Part model, mm, in its own coordinate system. A direction names the side the tool comes from. Round coordinates to 2 decimals unless told otherwise and drop trailing zeros. Write each loop counter-clockwise with the first axis right and the second up, starting at its lowest first coordinate (ties: lowest second). Pieces come first, ordered by that corner, then holes. Notation, with made-up numbers: M 28,19 L 32,19 A27 cw 32,44 Z; hole C 14.5,12.5 d7. An arc over 180 degrees is marked long. Answer as a JSON object with one key per item and string values. Group by question number.
1. Band-saw the part on B-B, the plane y = -76. Write the cut outline in (x, z), plus the area to 3 significant figures.
2. Two-plate mould, pull along Z, no slides. Class faces 1 (the face through (-557.59, 0.09, -6.7)), 2 (the face through (6, -2, 6.35)), 3 (the face through (-529.17, 0.089, 19.663)): +Z half, -Z half, draft (parallel to the pull), parting line (faces both ways), or undercut.
3. Drop flat-ended pins along their axis: pin 1 (6.5 mm diameter, centred on y = -54.5, z = 2.5, fed in from -X); pin 2 (6 mm diameter, centred on x = -98, z = 6.5, fed in from +Y); pin 3 (4 mm diameter, centred on x = 4, y = 30, fed in from +Z). Give the stop position or say it passes through.
4. Band-saw the part on C-C, the plane x = -351.5. Write the cut outline in (y, z).
5. Drill centre lines: line 1 (Z direction, x = -133.5, y = 1); line 2 (Z direction, x = -244.5, y = -3.5). Where is each one in solid material? Low to high. Write a range as from..to.
6. Band-saw the part on A-A, the plane x = -513. Count the separate pieces of the cut face and the enclosed holes in it, plus the area to 3 significant figures.
7. Which spindle directions (+Z, -Z, +X, -X, +Y, -Y) get a long thin tool onto all of the face, cutting with end or side? Do faces 4 (the face through (-521, -6.35, 25)), 5 (the face through (-521, 6.35, 25)), 6 (the face through (-528.791, 0.089, 85.426)). Say none if no direction does.
from build123d import *

# Parameters (mm, degrees)
F0_W      = 254
F0_H      = 12.7
F1_DEPTH  = 12.7
F3_DEPTH  = 558.8
F4_R      = 7.62
F6_DEPTH  = 12.7
F7_W      = 101.6
F7_H      = 12.7
F8_DEPTH  = 2.54
F10_DEPTH = 50.8


with BuildPart() as f1:
    # F0 (on Right) → F1 (new body)
    with BuildSketch(Plane.YZ):
        Rectangle(F0_W, F0_H)
    extrude(amount=F1_DEPTH)

    # F2 (on face) → F3 (join)
    with BuildSketch(Plane(origin=(0, 0, 0), x_dir=(0, -1, 0), z_dir=(-1, 0, 0))):
        with BuildLine():
            ThreePointArc((-6.84e-08, -6.35), (4.4901280364, -4.4901280847), (6.35, 0))
            ThreePointArc((6.35, 0), (4.4901280521, 4.4901280689), (-2.37e-08, 6.35))
            ThreePointArc((-2.37e-08, 6.35), (-6.35, 2.23e-08), (-6.84e-08, -6.35))
        make_face()
    extrude(amount=F3_DEPTH)

    # F4
    f4_edges = [f1.edges().sort_by_distance(p)[0] for p in [
        (6.35, -127, -6.35),
        (6.35, 127, -6.35),
    ]]
    fillet(f4_edges, radius=F4_R)

    # F5 (on Front) → F6 (cut, symmetric)
    with BuildSketch(Plane.XZ):
        Polygon((-541.0905659676, 6.7056384869), (-558.8, 6.7056384869), (-558.8, -7.6832813211), align=None)
    extrude(amount=F6_DEPTH, both=True, mode=Mode.SUBTRACT)

    # F7 (on face) → F8 (join)
    with BuildSketch(Plane(origin=(-218.4449745832, 0, 268.8552663249), x_dir=(0.7761139002, 0, 0.630592748), z_dir=(-0.630592748, 0, 0.7761139002))):
        with Locations((-388.1941093914, 0)):
            Rectangle(F7_W, F7_H)
    extrude(amount=F8_DEPTH)

    # F9 (on face) → F10 (join)
    with BuildSketch(Plane(origin=(-220.0466801631, 0, 270.8265956315), x_dir=(0.7761139002, 0, 0.630592748), z_dir=(-0.630592748, 0, 0.7761139002))):
        with BuildLine():
            ThreePointArc((-356.4441093914, -6.35), (-351.9539813308, -4.4901280605), (-350.0941093914, 0))
            ThreePointArc((-350.0941093914, 0), (-351.9539813308, 4.4901280605), (-356.4441093914, 6.35))
            ThreePointArc((-356.4441093914, 6.35), (-362.7941093914, 0), (-356.4441093914, -6.35))
        make_face()
    extrude(amount=F10_DEPTH)


solid = f1.part
Worked answers:
{
 "1": {"outline": "M 0,-6.35 L 12.7,-6.35 L 12.7,6.35 L 0,6.35 Z", "area": "161 mm^2"},
 "2": {"face 1": "-Z half", "face 2": "+Z half", "face 3": "undercut"},
 "3": {"pin 1": "stops at x = 0", "pin 2": "stops at y = 5.3", "pin 3": "stops at z = 6.35"},
 "4": {"outline": "C 0,0 d12.7"},
 "5": {"line 1": "z = -6.27..6.27", "line 2": "z = -5.3..5.3"},
 "6": {"separate pieces": "3", "enclosed holes": "0", "area": "369 mm^2"},
 "7": {"face 4": "+Z, -Z, -X, -Y", "face 5": "+Z, -Z, -X, +Y", "face 6": "+Z, -X, +Y, -Y"}
}
